```python
from build123d import *

# Parameters (mm, degrees)
SKETCH1_W           = 10
SKETCH1_H           = 25
BOSS_EXTRUDE1_DEPTH = 410
SKETCH2_W           = 9
SKETCH2_H           = 23
CUT_EXTRUDE1_DEPTH  = 410
CUT_EXTRUDE2_DEPTH  = 410
CUT_EXTRUDE3_DEPTH  = 410
CUT_EXTRUDE4_DEPTH  = 410


with BuildPart() as part:
    # Sketch1 → Boss-Extrude1 (new body)
    with BuildSketch(Plane(origin=(0, 0, 0), x_dir=(1, 0, 0), z_dir=(0, 1, 0))):
        with Locations((5, -12.5)):
            Rectangle(SKETCH1_W, SKETCH1_H)
    extrude(amount=BOSS_EXTRUDE1_DEPTH)

    # Sketch2 → Cut-Extrude1 (cut)
    with BuildSketch(Plane(origin=(0, 410, 0), x_dir=(1, 0, 0), z_dir=(0, 1, 0))):
        with Locations((5.5, -12.5)):
            Rectangle(SKETCH2_W, SKETCH2_H)
    extrude(amount=-CUT_EXTRUDE1_DEPTH, mode=Mode.SUBTRACT)

    # Sketch3 → Cut-Extrude2 (cut)
    with BuildSketch(Plane.ZY):
        with BuildLine():
            Line((11.5, 391), (13.5, 391))
            ThreePointArc((13.5, 391), (14.5, 390), (13.5, 389))
            Line((13.5, 389), (11.5, 389))
            ThreePointArc((11.5, 389), (10.5, 390), (11.5, 391))
        make_face()
    extrude(amount=-CUT_EXTRUDE2_DEPTH, mode=Mode.SUBTRACT)

    # Sketch3<3> → Cut-Extrude3 (cut)
    with BuildSketch(Plane.ZY):
        with BuildLine():
            Line((14.5, 370), (14.5, 362))
            ThreePointArc((14.5, 362), (12.5, 360), (10.5, 362))
            Line((10.5, 362), (10.5, 370))
            ThreePointArc((10.5, 370), (12.5, 372), (14.5, 370))
        make_face()
    extrude(amount=-CUT_EXTRUDE3_DEPTH, mode=Mode.SUBTRACT)

    # Sketch3<4> → Cut-Extrude4 (cut)
    with BuildSketch(Plane.ZY):
        with BuildLine():
            Line((11.5, 344.4), (13.5, 344.4))
            ThreePointArc((13.5, 344.4), (15.9, 342), (13.5, 339.6))
            Line((13.5, 339.6), (11.5, 339.6))
            ThreePointArc((11.5, 339.6), (9.1, 342), (11.5, 344.4))
        make_face()
    extrude(amount=-CUT_EXTRUDE4_DEPTH, mode=Mode.SUBTRACT)


solid = part.part
```
Input: part model. Units: mm. Frame: model coordinates. A direction names the side the tool comes from. Coordinates: 2 decimals unless noted, no trailing zeros. Write each loop counter-clockwise with the first axis right and the second up, starting at its lowest first coordinate (ties: lowest second). Pieces come first, ordered by that corner, then holes. Notation, with made-up numbers: (50, 2.5) - (64, 2.5) arc R20 ccw to (64, 33.5) - close; hole circle Ø8 at (-6, 52). An arc over 180 degrees is marked (long way). Put each result on its own line as item: value. Start each with the question number.
1) Cut plane A-A (x = 7.75). Return the cut outline in (y, z).
2) Cut plane B-B (y = 126). Return the cut outline in (x, z).
3) Contact query for flat-ended pins moving along their axis: pin 1 (4 mm diameter, centred on y = 367.5, z = 18, fed in from +X); pin 2 (1.1 mm diameter, centred on x = 0.5, z = 12.5, fed in from -Y). Output: stop coordinate, or through.
4) Mould query, pull axis Z, two halves, no side actions, for faces 3 (the face through (5, 208, 24)), 4 (the face through (5, 202, 0)), 5 (the face through (0, 202, 13)), 6 (the face through (5, 208, 1)). Classes: pulls with the +Z half, pulls with the -Z half, needs draft (parallel to the pull), parting line crosses it, or undercut.
5) Cut plane C-C (z = 5). Return the cut outline in (x, y), plus the area to 3 significant figures.
6) Ray query, L1, parallel to Z at x = 7.5, y = 86; L2, parallel to X at y = 160, z = 20. Return the intervals inside material, ascending.
7) Reachability of faces 1 (the face through (1, 208, 13)), 2 (the face through (0.5, 0, 12.4)) from +Z, -Z, +X, -X, +Y, -Y: full face, straight path, thin tool, end or side. Return the list, or none.
Resolved:
1. outline: (0, 0) - (410, 0) - (410, 1) - (0, 1) - close; (0, 24) - (410, 24) - (410, 25) - (0, 25) - close
2. outline: (0, 0) - (10, 0) - (10, 1) - (1, 1) - (1, 24) - (10, 24) - (10, 25) - (0, 25) - close
3. pin 1: stops at x = 1
3. pin 2: stops at y = 0
4. face 3: undercut
4. face 4: pulls with the -Z half
4. face 5: needs draft
4. face 6: undercut
5. outline: (0, 0) - (1, 0) - (1, 410) - (0, 410) - close
5. area: 410 mm2
6. L1: z = 0 to 1, 24 to 25
6. L2: x = 0 to 1
7. face 1: +X, +Y, -Y
7. face 2: +Z, -Z, +X, -X, -Y
